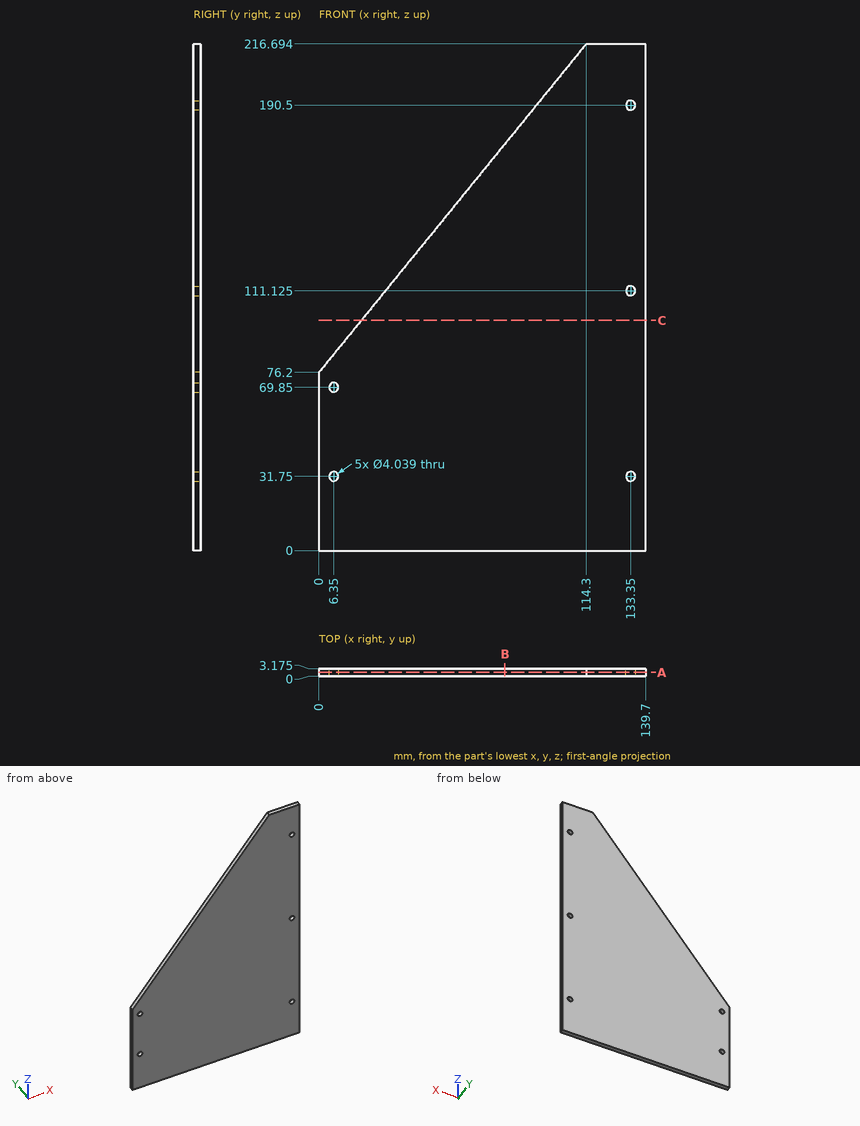
The drawing under review shows one solid part. Ordinate dimensions are in mm from its lowest x, y, z. Round coordinates to 2 decimals unless told otherwise and drop trailing zeros. Write each loop counter-clockwise with the first axis right and the second up, starting at its lowest first coordinate (ties: lowest second). Pieces come first, ordered by that corner, then holes. Notation, with made-up numbers: (47, 8.5) -> (67, 8.5) arc R23 ccw to (67, 47.5) -> close; hole circle Ø8 at (65, 19.5). An arc over 180 degrees is marked (long way). Put each result on its own line as item: value.
Q1. Consider section A-A on y = 1.55. Give the number of separate pieces and of enclosed holes in the cut face, and give its area (3 significant figures).
Determined:
separate pieces: 1
enclosed holes: 5
area: 22,200 mm^2
Q2. Consider section B-B on x = 79.5. State the section outline as (y, z) points (1 decimal), and give its area (3 significant figures).
Determined:
outline: (0, 0) -> (3.2, 0) -> (3.2, 173.9) -> (0, 173.9) -> close
area: 552 mm^2
Q3. To check wall thickness, follow L1, parallel to Z at x = 133.35, y = 1.8 (1 decimal); L2, parallel to Z at x = 6.35, y = 2.35 (1 decimal); L3, parallel to X at y = 2.55, z = 32.5 (1 decimal). State the ranges of each line that lie inside material, in increasing order. Write a range as [from, to].
Determined:
L1: z = [0, 29.7], [33.8, 109.1], [113.1, 188.5], [192.5, 216.7]
L2: z = [0, 29.7], [33.8, 67.8], [71.9, 84]
L3: x = [0, 4.5], [8.2, 131.5], [135.2, 139.7]
Q4. Clearance check with flat-ended pins moving along their axes: pin 1 Ø4.5 at (x, z) = (6.35, 69.85) entering from -Y; pin 2 Ø1 at (y, z) = (1.5, 127.5) entering from -X; pin 3 Ø1 at (y, z) = (0.5, 168.5) entering from -X (1 decimal). State where each tip first meets the part, or that it passes through.
Determined:
pin 1: stops at y = 0
pin 2: stops at x = 41.33
pin 3: stops at x = 74.7
Q5. Consider section C-C on z = 98.5. State the section outline as (x, y) points (1 decimal), and give its area (3 significant figures).
Determined:
outline: (18.1, 0) -> (139.7, 0) -> (139.7, 3.2) -> (18.1, 3.2) -> close
area: 386 mm^2
